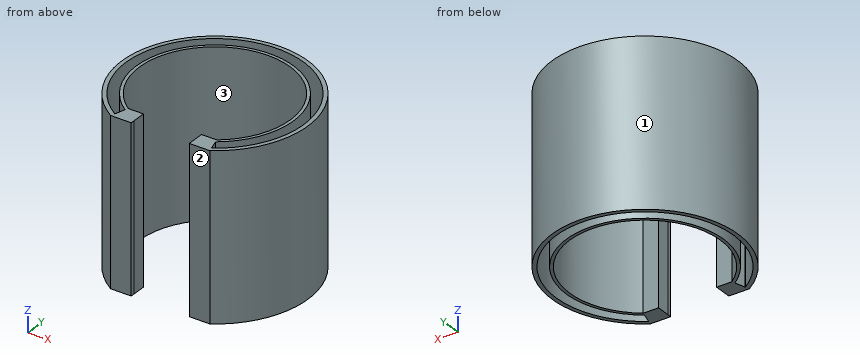
from build123d import *

# Parameters (mm, degrees)
F1_DEPTH = 160
F3_DEPTH = 160
F4_W     = 56.415766
F4_H     = 160
F5_DEPTH = 4
F7_DEPTH = 160


with BuildPart() as f1:
    # F0 (on Top) → F1 (new body)
    with BuildSketch(Plane.XY):
        with BuildLine():
            Line((-48.207883, -76), (48.207883, -76))
            ThreePointArc((48.207883, -76), (0, 90), (-48.207883, -76))
        make_face()
    extrude(amount=F1_DEPTH)

    # F2 (on face) → F3 (cut, through all)
    with BuildSketch(Plane.XY.offset(160)):
        with BuildLine():
            Line((-47.031904, -72), (47.031904, -72))
            ThreePointArc((47.031904, -72), (0, 86), (-47.031904, -72))
        make_face()
    extrude(amount=-F3_DEPTH, mode=Mode.SUBTRACT)

    # F4 (on face) → F5 (cut, through all)
    with BuildSketch(Plane.XZ.offset(76)):
        with Locations((0, 80)):
            Rectangle(F4_W, F4_H)
    extrude(amount=-F5_DEPTH, mode=Mode.SUBTRACT)

    # F6 (on Top) → F7 (join)
    with BuildSketch(Plane.XY):
        with BuildLine():
            Line((46.919916, -72.018087), (43.954522, -62))
            ThreePointArc((43.954522, -62), (0, 76), (-43.954522, -62))
            Line((-43.954522, -62), (-46.919916, -72.018087))
            Line((-46.919916, -72.018087), (-28.151507, -72.018087))
            Line((-28.151507, -72.018087), (-28.207883, -59))
            Line((-28.207883, -59), (-42.988371, -59))
            ThreePointArc((-42.988371, -59), (0, 73), (42.988371, -59))
            Line((42.988371, -59), (28.207883, -59))
            Line((28.207883, -59), (28.151507, -72.018087))
            Line((28.151507, -72.018087), (46.919916, -72.018087))
        make_face()
    extrude(amount=F7_DEPTH)


solid = f1.part
Design review of the part built by this model. Coordinates are the model's own, in mm. Face numbers are marked on the shaded views. Coordinates: 2 decimals unless noted, no trailing zeros. Order: outer loops, then holes, each group sorted by start corner. A loop starts at its lowest first (then second) coordinate and runs counter-clockwise, first axis right, second up. Notation, with made-up numbers: M 57,50 L 100,50 A15 cw 100,67 Z; hole C 70.5,-0.5 d8. An arc over 180 degrees is marked long. Use a Markdown table: item, result.
(1) Add section A-A (x = 0). Give the boundary of the cut face in (y, z), then the cut area to 3 significant figures.
Worked answers:
| item | result |
|---|---|
| outline | M 73,0 L 76,0 L 76,160 L 73,160 Z; M 86,0 L 90,0 L 90,160 L 86,160 Z |
| area | 1,120 mm2 |
(2) Draft analysis for pull direction Y (two halves, no side actions). For the marked faces 1, 2 and 3, state which applies: released by +Y, released by -Y, zero draft, split by the parting line, or undercut.
Worked answers:
| item | result |
|---|---|
| face 1 | split by the parting line |
| face 2 | released by -Y |
| face 3 | undercut |
(3) Add section B-B (y = 0). Give the boundary of the cut face in (x, z).
Worked answers:
| item | result |
|---|---|
| outline | M -90,0 L -86,0 L -86,160 L -90,160 Z; M -76,0 L -73,0 L -73,160 L -76,160 Z; M 73,0 L 76,0 L 76,160 L 73,160 Z; M 86,0 L 90,0 L 90,160 L 86,160 Z |
(4) For P1, Ø2, axis at y = -74, z = 56, coming from the -X side; P2, Ø6, axis at x = -55.5, z = 90.5, coming from the +Y side; P3, Ø3, axis at x = -49, y = -50.5, coming from the -Z side; P4, Ø6, axis at y = 12.5, z = 42.5, coming from the +X side, all flat-tipped, find the tip position at first contact; note any pin that passes through.
Worked answers:
| item | result |
|---|---|
| P1 | stops at x = -52.64 |
| P2 | stops at y = 73.1 |
| P3 | passes through |
| P4 | stops at x = 89.5 |
(5) Add section D-D (y = 79). Give the boundary of the cut face in (x, z).
Worked answers:
| item | result |
|---|---|
| outline | M -43.12,0 L -33.99,0 L -33.99,160 L -43.12,160 Z; M 33.99,0 L 43.12,0 L 43.12,160 L 33.99,160 Z |
(6) Add section C-C (z = 71.5). Give the boundary of the cut face in (x, y).
Worked answers:
| item | result |
|---|---|
| outline | M -48.21,-76 L -28.21,-76 L -28.21,-72.02 L -28.15,-72.02 L -28.21,-59 L -42.99,-59 A73 cw long 42.99,-59 L 28.21,-59 L 28.15,-72.02 L 28.21,-72.02 L 28.21,-76 L 48.21,-76 A90 ccw long Z; hole M -47.03,-72 L -46.91,-72 L -43.95,-62 A76 cw long 43.95,-62 L 46.91,-72 L 47.03,-72 A86 ccw long Z |
(7) Wall thickness on probe 1 along X at (y, z) = (0, 115); probe 2 along Y at (x, z) = (55, 53); probe 3 along Y at (x, z) = (32, 73): over which ranges is each line inside the solid? List them lowest first.
Worked answers:
| item | result |
|---|---|
| probe 1 | x = -90 to -86, -76 to -73, 73 to 76, 86 to 90 |
| probe 2 | y = -71.24 to -66.11, -52.45 to -48, 48 to 52.45, 66.11 to 71.24 |
| probe 3 | y = -76 to -59, 65.61 to 68.93, 79.82 to 84.12 |
